Geometry check sheet. Reference: the model listing, model coordinates, mm. A direction names the side the tool comes from. Round coordinates to 2 decimals unless told otherwise and drop trailing zeros. Write each loop counter-clockwise with the first axis right and the second up, starting at its lowest first coordinate (ties: lowest second). Pieces come first, ordered by that corner, then holes. Notation, with made-up numbers: (43.25, -23) - (67.25, -23) arc R14 ccw to (67.25, -11) - close; hole circle Ø4 at (83, 7). An arc over 180 degrees is marked (long way). Return JSON: item names as keys, results as strings.
```python
from build123d import *

# Parameters (mm, degrees)
F0_W      = 65
F0_H      = 18
F1_DEPTH  = 17
F2_W      = 24
F2_H      = 18
F3_DEPTH  = 6
F4_R      = 2.75
F5_DEPTH  = 17
F7_DEPTH  = 10
F8_W      = 65
F8_H      = 1.2
F9_DEPTH  = 0.45
F11_DEPTH = 1.2
F13_DEPTH = 6
F14_R     = 1.5
F15_DEPTH = 11
F16_R     = 1.5
F17_DEPTH = 10
F18_R     = 1.5
F19_DEPTH = 10


with BuildPart() as f1:
    # F0 (on Front) → F1 (new body)
    with BuildSketch(Plane.XZ):
        Rectangle(F0_W, F0_H)
    extrude(amount=-F1_DEPTH)

    # F2 (on face) → F3 (cut)
    with BuildSketch(Plane.XZ):
        Rectangle(F2_W, F2_H)
    extrude(amount=-F3_DEPTH, mode=Mode.SUBTRACT)

    # F4 (on face) → F5 (cut, through all)
    with BuildSketch(Plane.XZ):
        with Locations((-27.5, 2)):
            Circle(F4_R)
        with Locations((27.5, 2)):
            Circle(F4_R)
    extrude(amount=-F5_DEPTH, mode=Mode.SUBTRACT)

    # F6 (on face) → F7 (cut)
    with BuildSketch(Plane.XZ):
        with BuildLine():
            ThreePointArc((-14.5, 2), (-16, 3.5), (-17.5, 2))
            Line((-17.5, 2), (-16, 2))
            Line((-16, 2), (-14.5, 2))
        make_face()
        with BuildLine():
            ThreePointArc((17.5, 2), (16, 3.5), (14.5, 2))
            ThreePointArc((14.5, 2), (16, 0.5), (17.5, 2))
        make_face()
        with BuildLine():
            Line((-16, 2), (-17.5, 2))
            ThreePointArc((-17.5, 2), (-16, 0.5), (-14.5, 2))
            Line((-14.5, 2), (-16, 2))
        make_face()
    extrude(amount=-F7_DEPTH, mode=Mode.SUBTRACT)

    # F8 (on face) → F9 (cut)
    with BuildSketch(Plane.XZ):
        with Locations((0, -8.4)):
            Rectangle(F8_W, F8_H)
    extrude(amount=-F9_DEPTH, mode=Mode.SUBTRACT)

    # F10 (on face) → F11 (cut)
    with BuildSketch(Plane(origin=(0, 0, -9), x_dir=(1, 0, 0), z_dir=(0, 0, -1))):
        Polygon((-31.5, -0.45), (-32.5, -0.45), (-32.5, -0.626327), align=None)
        Polygon((32.5, -0.626327), (32.5, -0.45), (31.5, -0.45), align=None)
    extrude(amount=-F11_DEPTH, mode=Mode.SUBTRACT)

    # F12 (on face) → F13 (cut)
    with BuildSketch(Plane.XZ.offset(-6)):
        with BuildLine():
            ThreePointArc((-5.5, -1), (-5.93934, 0.06066), (-7, 0.5))
            ThreePointArc((-7, 0.5), (-8.06066, -2.06066), (-5.5, -1))
        make_face()
        with BuildLine():
            ThreePointArc((-5.5, 5.5), (-5.93934, 6.56066), (-7, 7))
            Line((-7, 7), (-7, 5.5))
            Line((-7, 5.5), (-7, 4))
            ThreePointArc((-7, 4), (-5.93934, 4.43934), (-5.5, 5.5))
        make_face()
        with BuildLine():
            Line((-7, 5.5), (-7, 7))
            ThreePointArc((-7, 7), (-8.5, 5.5), (-7, 4))
            Line((-7, 4), (-7, 5.5))
        make_face()
        with BuildLine():
            ThreePointArc((8.5, -1), (8.06066, 0.06066), (7, 0.5))
            ThreePointArc((7, 0.5), (5.93934, -2.06066), (8.5, -1))
        make_face()
        with BuildLine():
            ThreePointArc((8.5, 5.5), (8.06066, 6.56066), (7, 7))
            Line((7, 7), (7, 5.5))
            Line((7, 5.5), (7, 4))
            ThreePointArc((7, 4), (8.06066, 4.43934), (8.5, 5.5))
        make_face()
        with BuildLine():
            Line((7, 5.5), (7, 7))
            ThreePointArc((7, 7), (5.5, 5.5), (7, 4))
            Line((7, 4), (7, 5.5))
        make_face()
    extrude(amount=-F13_DEPTH, mode=Mode.SUBTRACT)

    # F14 (on face) → F15 (cut, through all)
    with BuildSketch(Plane.XZ.offset(-6)):
        with Locations((-8.75, -5.5)):
            Circle(F14_R)
        with Locations((-4.75, -5.5)):
            Circle(F14_R)
        with Locations((5.25, -5.5)):
            Circle(F14_R)
        with Locations((9.25, -5.5)):
            Circle(F14_R)
    extrude(amount=-F15_DEPTH, mode=Mode.SUBTRACT)

    # F16 (on face) → F17 (cut)
    with BuildSketch(Plane(origin=(0, 0, -9), x_dir=(1, 0, 0), z_dir=(0, 0, -1))):
        with BuildLine():
            ThreePointArc((29, -11), (27.5, -9.5), (26, -11))
            ThreePointArc((26, -11), (27.5, -12.5), (29, -11))
        make_face()
        with Locations((-27.5, -11)):
            Circle(F16_R)
    extrude(amount=-F17_DEPTH, mode=Mode.SUBTRACT)

    # F18 (on face) → F19 (cut)
    with BuildSketch(Plane.YZ.offset(32.5)):
        with Locations((7, 6)):
            Circle(F18_R)
    extrude(amount=-F19_DEPTH, mode=Mode.SUBTRACT)


solid = f1.part
```
(1) Material ranges on line 1 along Z through (x, y) = (-7, 10.65); line 2 along Y through (x, z) = (27.5, -2.25); line 3 along X through (y, z) = (10, 3.5), recorded low to high. Write a range as [from, to].
Response values:
{"line 1": "z = [-9, -2.5], [0.5, 4], [7, 9]", "line 2": "y = [0, 9.5], [12.5, 17]", "line 3": "x = [-32.5, -29.8], [-25.2, 25.2], [29.8, 32.5]"}
(2) Gauge pin test, flat ends, axial feed: pin 1 (9 mm diameter, centred on x = 4, z = 1, fed in from -Y); pin 2 (0.5 mm diameter, centred on x = 20, y = 0, fed in from -Z); pin 3 (2.5 mm diameter, centred on x = 9.25, z = -5.5, fed in from -Y); pin 4 (1.5 mm diameter, centred on x = -7.5, z = 5.5, fed in from -Y). Record the tip position at first contact, or that the pin passes through.
Response values:
{"pin 1": "stops at y = 6", "pin 2": "stops at z = -7.8", "pin 3": "passes through", "pin 4": "stops at y = 12"}
(3) Section check D-D, the plane y = 7. Give the number of separate pieces and of enclosed holes in the cut face, plus the area to 3 significant figures.
Response values:
{"separate pieces": "1", "enclosed holes": "11", "area": "1,020 mm^2"}
(4) Section check B-B, the plane y = 2.25. Enter the section's corners in (x, z).
Response values:
{"outline": "(-32.5, -9) - (-12, -9) - (-12, 9) - (-32.5, 9) - close; (12, -9) - (32.5, -9) - (32.5, 9) - (12, 9) - close; hole circle Ø5.5 at (-27.5, 2); hole circle Ø3 at (-16, 2); hole circle Ø3 at (16, 2); hole circle Ø5.5 at (27.5, 2)"}
(5) Access from +Z, -Z, +X, -X, +Y, -Y to the whole of each face (thin tool, end or side, straight path). Record for faces 1 (the face through (-27.858, 8.381, 4.727)), 2 (the face through (-22, 0.45, -8)), 3 (the face through (22.5, 7, 6)), 4 (the face through (12, 3, 0)), 5 (the face through (16, 10, 2)).
Response values:
{"face 1": "+Y, -Y", "face 2": "-Z, +X, -X, -Y", "face 3": "+X", "face 4": "+Z, -Z, -Y", "face 5": "-Y"}
(6) Section check C-C, the plane x = -28. Enter the section's corners in (y, z), plus the area to 3 significant figures.
Response values:
{"outline": "(0, -7.8) - (0.45, -7.8) - (0.45, -9) - (9.59, -9) - (9.59, -0.7) - (0, -0.7) - close; (0, 4.7) - (17, 4.7) - (17, 9) - (0, 9) - close; (12.41, -9) - (17, -9) - (17, -0.7) - (12.41, -0.7) - close", "area": "190 mm^2"}
(7) Section check A-A, the plane x = -4.75. Enter the section's corners in (y, z), plus the area to 3 significant figures.
Response values:
{"outline": "(6, -9) - (17, -9) - (17, -7) - (6, -7) - close; (6, -4) - (17, -4) - (17, 9) - (6, 9) - close", "area": "165 mm^2"}
(8) Release check for a two-part mould opening along X. For faces 6 (the face through (-32.5, 8, 0)), 7 (the face through (-14.5, 4.93, 1.93)), 8 (the face through (-22, 0, 1)) record: pulls with the +X half, pulls with the -X half, needs draft (parallel to the pull), parting line crosses it, or undercut.
Response values:
{"face 6": "pulls with the -X half", "face 7": "undercut", "face 8": "needs draft"}
